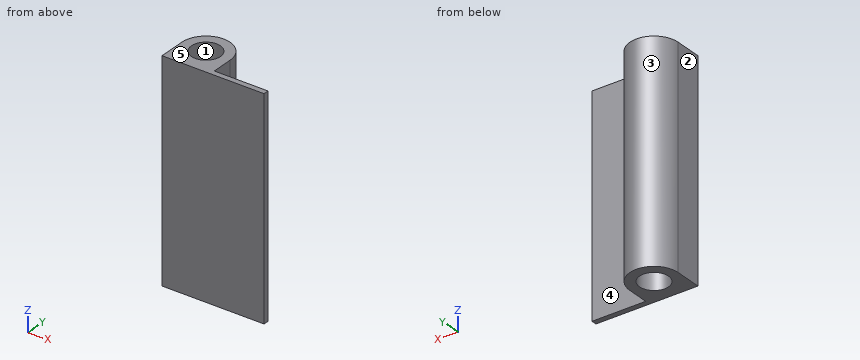
Autodesk Inventor part; units mm, degrees
ref_plane "YZ Plane" through (0, 0, 0) normal (1, 0, 0) x (0, 1, 0)
ref_plane "XZ Plane" through (0, 0, 0) normal (0, 1, 0) x (-1, 0, 0)
ref_plane "XY Plane" through (0, 0, 0) normal (0, 0, 1) x (1, 0, 0)
sketch "Sketch1" plane through (0, 0, 0) normal (0, 0, 1) x (1, 0, 0)
  line L0 (9, 0) -> (28, 0)
  line L1 (28, 0) -> (28, 1)
  line L2 (28, 1) -> (9, 1)
  line L3 (9, 1) -> (18, 1)
  line L4 (18, 1) -> (18, 5)
  line L5 (18, 5) -> (9, 5)
  line L6 (9, 5) -> (9, 1)
  circle A0 centre (13.5, 5) radius 4.5
  circle A1 centre (13.5, 5) radius 2.5
  line L7 (9, 1) -> (9, 0)
  point P0 (0, 0)
  point P1 (28, 0.5)
  point P2 (18, 1)
  point P3 (11.4384, 1)
  point P4 (15.5616, 1)
  dimension "d1" = 1
  dimension "d2" = 5
  dimension "d3" = 5
  dimension "d4" = 2
  dimension "d5" = 10
  dimension "d11" = 9
extrude "Extrusion1" add sketch "Sketch1" along normal blind 40 contours L7 L2 A0 L1 L0 | L6 A0 L2 | A0 L5 A1 L2 | L2 A0 | A0 L5 A1 | L2 A0 L4
thicken "Thicken1" operation cut thickness 0.2 both sides no extend neighbours no toward (0.9870503, -0.1604113, 0) faces at (15.9676, 4.599, 26.6667)
properties part number "LI0017-LATCH BARREL"
Part model, mm, in its own coordinate system. Face numbers are marked on the shaded views. A direction names the side the tool comes from. Coordinates: 2 decimals unless noted, no trailing zeros. Order: outer loops, then holes, each group sorted by start corner. A loop starts at its lowest first (then second) coordinate and runs counter-clockwise, first axis right, second up.
(1) Slice it at B-B, the plane y = 3.75. Write the cut outline in (x, z).
Check sheet entries:
outline: (9, 0) - (11.11, 0) - (11.11, 40) - (9, 40) - close; (15.89, 0) - (18, 0) - (18, 40) - (15.89, 40) - close
(2) Pin check, flat tips, straight feed: pin 1 Ø4 at (x, z) = (19.5, 7.5) entering from +Y; pin 2 Ø3 at (x, z) = (21, 24) entering from +Y; pin 3 Ø2 at (y, z) = (4, 17.5) entering from +X. Stop position of each tip, or through.
Check sheet entries:
pin 1: stops at y = 7.06
pin 2: stops at y = 1
pin 3: stops at x = 18
(3) Pull direction Y, two halves, no side cores. Call the marked faces 1, 2 and 3: pulls with the +Y half, pulls with the -Y half, needs draft (parallel to the pull), parting line crosses it, or undercut.
Check sheet entries:
face 1: undercut
face 2: needs draft
face 3: pulls with the +Y half
(4) Tool access for the marked faces 4 and 5: list every direction of +Z, -Z, +X, -X, +Y, -Y with a clear straight run to the whole face (end or side of a thin tool).
Check sheet entries:
face 4: +Z, -Z, +X, +Y
face 5: +Z, +X, -X, +Y, -Y
(5) Slice it at A-A, the plane x = 13.5. Write the cut outline in (y, z).
Check sheet entries:
outline: (0, 0) - (2.3, 0) - (2.3, 40) - (0, 40) - close; (7.7, 0) - (9.5, 0) - (9.5, 40) - (7.7, 40) - close
(6) Probe L1, parallel to X at y = 5, z = 19; L2, parallel to Y at x = 13.5, z = 20; L3, parallel to Y at x = 22.5, z = 17. List the from-to ranges inside material, lowest first.
Check sheet entries:
L1: x = 9 to 10.8, 16.2 to 18
L2: y = 0 to 2.3, 7.7 to 9.5
L3: y = 0 to 1
(7) Slice it at C-C, the plane z = 18. Write the cut outline in (x, y).
Check sheet entries:
outline: (9, 0) - (28, 0) - (28, 1) - (18, 1) - (18, 5) arc R4.5 ccw to (9, 5) - close; hole circle Ø5.4 at (13.5, 5)
(8) Slice it at D-D, the plane x = 23.75. Write the cut outline in (y, z).
Check sheet entries:
outline: (0, 0) - (1, 0) - (1, 40) - (0, 40) - close
